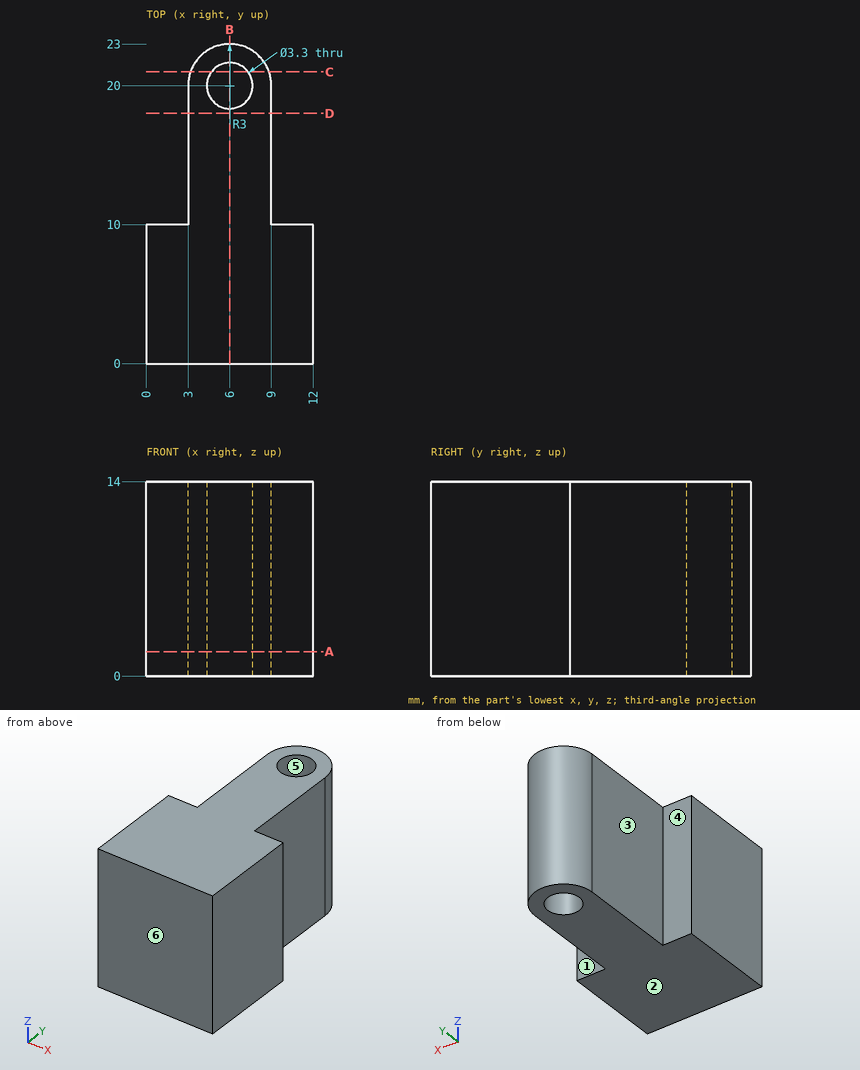
Check sheet for the drawn part. Datum: minimum x, y, z corner. Units: mm. A direction names the side the tool comes from. Round coordinates to 2 decimals unless told otherwise and drop trailing zeros. Order: outer loops, then holes, each group sorted by start corner. A loop starts at its lowest first (then second) coordinate and runs counter-clockwise, first axis right, second up.
1. Section check A-A on z = 1.75. Record the cut outline in (x, y).
Final values:
outline: (0, 0) - (12, 0) - (12, 10) - (9, 10) - (9, 20) arc R3 ccw to (3, 20) - (3, 10) - (0, 10) - close; hole circle Ø3.3 at (6, 20)
2. Access from +Z, -Z, +X, -X, +Y, -Y to the whole of each face (thin tool, end or side, straight path). Record for the marked faces 1 and 2.
Final values:
face 1: +Z, -Z, +X, +Y
face 2: -Z, +X, -X, +Y, -Y
3. Section check D-D on y = 18. Record the cut outline in (x, z), then the cut area to 3 significant figures.
Final values:
outline: (3, 0) - (9, 0) - (9, 14) - (3, 14) - close
area: 84.0 mm2
4. Section check C-C on y = 21. Record the cut outline in (x, z).
Final values:
outline: (3.17, 0) - (4.69, 0) - (4.69, 14) - (3.17, 14) - close; (7.31, 0) - (8.83, 0) - (8.83, 14) - (7.31, 14) - close
5. Section check B-B on x = 6. Record the cut outline in (y, z).
Final values:
outline: (0, 0) - (18.35, 0) - (18.35, 14) - (0, 14) - close; (21.65, 0) - (23, 0) - (23, 14) - (21.65, 14) - close
6. Release check for a two-part mould opening along Y. For the marked faces 3, 4, 5 and 6 record: +Y half, -Y half, draft (parallel to the pull), parting line (faces both ways), or undercut.
Final values:
face 3: draft
face 4: +Y half
face 5: undercut
face 6: -Y half
7. Go/stop test with flat-tipped pins: P1, Ø5, axis at y = 13, z = 10, coming from the +X side; P2, Ø3, axis at x = 6, y = 20, coming from the +Z side; P3, Ø4, axis at y = 20.5, z = 10.5, coming from the -X side; P4, Ø1.5, axis at x = 10.5, z = 4, coming from the +Y side. Record where each tip stops, or that it passes through.
Final values:
P1: stops at x = 9
P2: passes through
P3: stops at x = 3
P4: stops at y = 10
8. Thickness scan on L1, parallel to Y at x = 6, z = 5.5; L2, parallel to Y at x = 10.5, z = 7.75; L3, parallel to X at y = 17.5, z = 7.25. Record the ranges inside material, lowest first.
Final values:
L1: y = 0 to 18.35, 21.65 to 23
L2: y = 0 to 10
L3: x = 3 to 9
